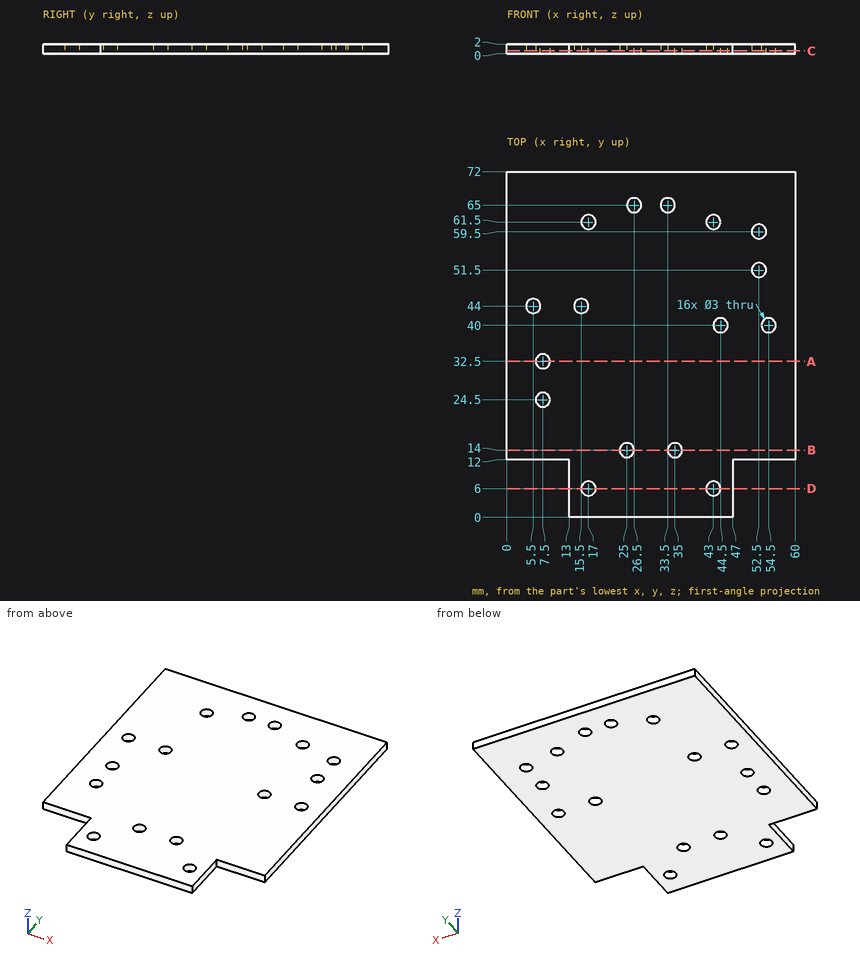
Geometry check sheet. Reference: drawing and pictorial views, mm from the part's lowest x, y, z. Give positions to 0.01 mm unless a question says otherwise; leave off trailing zeros. Order: outer loops, then holes, each group sorted by start corner. A loop starts at its lowest first (then second) coordinate and runs counter-clockwise, first axis right, second up. Notation, with made-up numbers: M -23,23 L 4,23 A23 cw 4,42 Z; hole C 67.25,6 d11. An arc over 180 degrees is marked long. Use one line per item in the form item = value. Start each with the question number.
Q1. Section check C-C (z = 0.55). Count the separate pieces of the cut face and the enclosed holes in it, then the cut area to 3 significant figures.
Q2. Scan lines: line 1 along X through (y, z) = (32.5, 0.85); line 2 along Y through (x, z) = (9.5, 1.4); line 3 along X through (y, z) = (32, 0.5). Record each from-to range of solid material in increasing order. Write a range as [from, to].
Q3. Section check B-B (y = 14). Enter the section's corners in (x, z), then the cut area to 3 significant figures.
Q4. Section check D-D (y = 6). Enter the section's corners in (x, z).
Q5. Section check A-A (y = 32.5). Enter the section's corners in (x, z).
Q6. Go/stop test with flat-tipped pins: pin 1 Ø10 at (x, y) = (38, 32) entering from -Z; pin 2 Ø2.5 at (x, y) = (15.5, 44) entering from +Z; pin 3 Ø0.6 at (y, z) = (7.5, 1.5) entering from +X; pin 4 Ø1 at (x, z) = (5.5, 0.5) entering from -Y. Record where each tip stops, or that it passes through.
Evaluation:
q1.separate_pieces = 1
q1.enclosed_holes = 16
q1.area = 3,890 mm2
q2.line_1 = [0, 6], [9, 60]
q2.line_2 = [12, 72]
q2.line_3 = [0, 6.09], [8.91, 60]
q3.outline = M 0,0 L 23.5,0 L 23.5,2 L 0,2 Z; M 26.5,0 L 33.5,0 L 33.5,2 L 26.5,2 Z; M 36.5,0 L 60,0 L 60,2 L 36.5,2 Z
q3.area = 108 mm2
q4.outline = M 13,0 L 15.5,0 L 15.5,2 L 13,2 Z; M 18.5,0 L 41.5,0 L 41.5,2 L 18.5,2 Z; M 44.5,0 L 47,0 L 47,2 L 44.5,2 Z
q5.outline = M 0,0 L 6,0 L 6,2 L 0,2 Z; M 9,0 L 60,0 L 60,2 L 9,2 Z
q6.pin_1 = 0
q6.pin_2 = through
q6.pin_3 = 47
q6.pin_4 = 12
